Geometry check sheet. Reference: the model listing, model coordinates, mm. A direction names the side the tool comes from. Round coordinates to 2 decimals unless told otherwise and drop trailing zeros. Order: outer loops, then holes, each group sorted by start corner. A loop starts at its lowest first (then second) coordinate and runs counter-clockwise, first axis right, second up. Notation, with made-up numbers: (-37.75, 2) - (2.25, 2) arc R25 ccw to (2.25, 16) - close; hole circle Ø7 at (31, 60). An arc over 180 degrees is marked (long way). Return JSON: item names as keys, results as strings. Group by question number.
Q1. Sectioned sample at A-A, the plane y = 2.5. Give the number of separate pieces and of enclosed holes in the cut face, then the cut area to 3 significant figures.
Q2. Material ranges on line 1 along Z through (x, y) = (-15.45, 3.5); line 2 along X through (y, z) = (2.75, 38); line 3 along Z through (x, y) = (-17, 2), recorded low to high.
Q3. Draft check along X on faces 1 (the flat face through (6.7, 3, 38)), 2 (the flat face through (9, 6.7, 37)), 3 (the flat face through (11.7, 3, 38)). Enter one of: pulls with the +X half, pulls with the -X half, needs draft (parallel to the pull), parting line crosses it, or undercut.
Q4. Sectioned sample at B-B, the plane x = -15.45. Record the cut outline in (y, z), then the cut area to 3 significant figures.
Q5. Tool access check on faces 4 (the flat face through (-6.7, 3, 37)), 5 (the cylindrical face through (-14.91, 3.45, 12.56)). Record the directions out of +Z, -Z, +X, -X, +Y, -Y that give a thin tool (end or side, any length) a straight path to the whole face; none if there is none.
Q6. Sectioned sample at D-D, the plane y = -2.25. Record the cut outline in (x, z).
Q7. Gauge pin test, flat ends, axial feed: pin 1 Ø15 at (x, z) = (-27.5, 49.5) entering from -Y; pin 2 Ø2 at (y, z) = (-3, 39.5) entering from +X; pin 3 Ø1 at (y, z) = (-2, 53.5) entering from +X; pin 4 Ø3 at (x, z) = (-32.95, 30) entering from -Y. Record the tip position at first contact, or that the pin passes through.
Q8. Sectioned sample at C-C, the plane z = 15. Record the cut outline in (x, y), then the cut area to 3 significant figures.
```python
from build123d import *

# Parameters (mm, degrees)
SKETCH3_W           = 5
SKETCH3_H           = 6.7
BOSS_EXTRUDE2_DEPTH = 75
SWEEP1_DEPTH        = 75
SKETCH8_W           = 5
SKETCH8_H           = 75
BOSS_EXTRUDE3_DEPTH = 6.7
SKETCH11_W          = 75
SKETCH11_H          = 6.6
BOSS_EXTRUDE4_DEPTH = 30
SKETCH12_R          = 2.5
CUT_EXTRUDE1_DEPTH  = 60


# Read off the part's stored shape, not the designer's step: Sweep1
with BuildPart() as part:
    # Sketch3 → Boss-Extrude2 (new body)
    with BuildSketch(Plane.XY):
        with Locations((-9.2, 3.35)):
            Rectangle(SKETCH3_W, SKETCH3_H)
    extrude(amount=BOSS_EXTRUDE2_DEPTH)

    # Sweep1 outline → Sweep1 (add)
    with BuildSketch(Plane.XY):
        with BuildLine():
            ThreePointArc((-11.7, 0), (0, -11.7), (11.7, 0))
            Line((11.7, 0), (6.7, 0))
            ThreePointArc((6.7, 0), (0, -6.7), (-6.7, 0))
            Line((-6.7, 0), (-11.7, 0))
        make_face()
    extrude(amount=SWEEP1_DEPTH)

    # Sketch8 → Boss-Extrude3 (add)
    with BuildSketch(Plane(origin=(0, 0, 0), x_dir=(1, 0, 0), z_dir=(0, 1, 0))):
        with Locations((9.2, -37.5)):
            Rectangle(SKETCH8_W, SKETCH8_H)
    extrude(amount=BOSS_EXTRUDE3_DEPTH)

    # Sketch11 → Boss-Extrude4 (add)
    with BuildSketch(Plane.ZY.offset(11.7)):
        with Locations((37.5, 3.4)):
            Rectangle(SKETCH11_W, SKETCH11_H)
    extrude(amount=BOSS_EXTRUDE4_DEPTH)

    # Sketch12 → Cut-Extrude1 (cut)
    with BuildSketch(Plane(origin=(0, 6.7, 0), x_dir=(1, 0, 0), z_dir=(0, 1, 0))):
        with Locations(Location((-15.45, -60, 0), (0, 0, 180))):
            Circle(SKETCH12_R)
        with Locations(Location((-15.45, -45, 0), (0, 0, 180))):
            Circle(SKETCH12_R)
        with Locations(Location((-32.95, -45, 0), (0, 0, 180))):
            Circle(SKETCH12_R)
        with Locations(Location((-32.95, -60, 0), (0, 0, 180))):
            Circle(SKETCH12_R)
        with Locations(Location((-15.45, -30, 0), (0, 0, 180))):
            Circle(SKETCH12_R)
        with Locations(Location((-32.95, -30, 0), (0, 0, 180))):
            Circle(SKETCH12_R)
        with Locations(Location((-15.45, -15, 0), (0, 0, 180))):
            Circle(SKETCH12_R)
        with Locations(Location((-32.95, -15, 0), (0, 0, 180))):
            Circle(SKETCH12_R)
    extrude(amount=-CUT_EXTRUDE1_DEPTH, mode=Mode.SUBTRACT)


solid = part.part
```
Reply:
{
 "1": {"separate pieces": "2", "enclosed holes": "8", "area": "2,840 mm^2"},
 "2": {"line 1": "0 to 12.5, 17.5 to 27.5, 32.5 to 42.5, 47.5 to 57.5, 62.5 to 75", "line 2": "-41.7 to -6.7, 6.7 to 11.7", "line 3": "0 to 13.04, 16.96 to 28.04, 31.96 to 43.04, 46.96 to 58.04, 61.96 to 75"},
 "3": {"face 1": "undercut", "face 2": "needs draft", "face 3": "pulls with the +X half"},
 "4": {"outline": "(0.1, 0) - (6.7, 0) - (6.7, 12.5) - (0.1, 12.5) - close; (0.1, 17.5) - (6.7, 17.5) - (6.7, 27.5) - (0.1, 27.5) - close; (0.1, 32.5) - (6.7, 32.5) - (6.7, 42.5) - (0.1, 42.5) - close; (0.1, 47.5) - (6.7, 47.5) - (6.7, 57.5) - (0.1, 57.5) - close; (0.1, 62.5) - (6.7, 62.5) - (6.7, 75) - (0.1, 75) - close", "area": "363 mm^2"},
 "5": {"face 4": "+Z, -Z, +Y", "face 5": "+Y, -Y"},
 "6": {"outline": "(-11.48, 0) - (-6.31, 0) - (-6.31, 75) - (-11.48, 75) - close; (6.31, 0) - (11.48, 0) - (11.48, 75) - (6.31, 75) - close"},
 "7": {"pin 1": "y = 0.1", "pin 2": "x = 11.53", "pin 3": "x = 11.6", "pin 4": "through"},
 "8": {"outline": "(-41.7, 0.1) - (-35.45, 0.1) - (-35.45, 6.7) - (-41.7, 6.7) - close; (-30.45, 0.1) - (-17.95, 0.1) - (-17.95, 6.7) - (-30.45, 6.7) - close; (-12.95, 0.1) - (-11.7, 0.1) - (-11.7, 0) arc R11.7 ccw to (11.7, 0) - (11.7, 6.7) - (6.7, 6.7) - (6.7, 0) arc R6.7 cw to (-6.7, 0) - (-6.7, 6.7) - (-12.95, 6.7) - close", "area": "344 mm^2"}
}
